Geometry: see drawing. Coordinates: mm, zero at the bounding-box minimum. A direction names the side the tool comes from. Coordinates: 2 decimals unless noted, no trailing zeros. Write each loop counter-clockwise with the first axis right and the second up, starting at its lowest first coordinate (ties: lowest second). Pieces come first, ordered by that corner, then holes. Notation, with made-up numbers: (-21, 9) - (-10, 9) arc R22 ccw to (-10, 41) - close; hole circle Ø9 at (12.5, -24.75). An arc over 180 degrees is marked (long way). One line per question, with ' | ' between items. Start each with the question number.
Q1. Contact query for flat-ended pins moving along their axis: P1, Ø2, axis at x = 5.5, z = 34, coming from the -Y side; P2, Ø1, axis at y = 4.5, z = 10, coming from the -X side. Output: stop coordinate, or through.
Q2. Cut plane A-A, the plane z = 9.5. Return loops of the section in (x, y).
Q3. Line query: line 1 (Z direction, x = 6.5, y = 2.25); line 2 (Y direction, x = 4.5, z = 2); line 3 (Y direction, x = 5, z = 3) (1 decimal). Output: solid intervals per line, ascending.
Q4. Access query for the marked faces 1 and 2. Directions: +Z, -Z, +X, -X, +Y, -Y. A direction counts if a zero-diameter tool reaches every point of the face in a straight line with its end or side. Return the directions, or none.
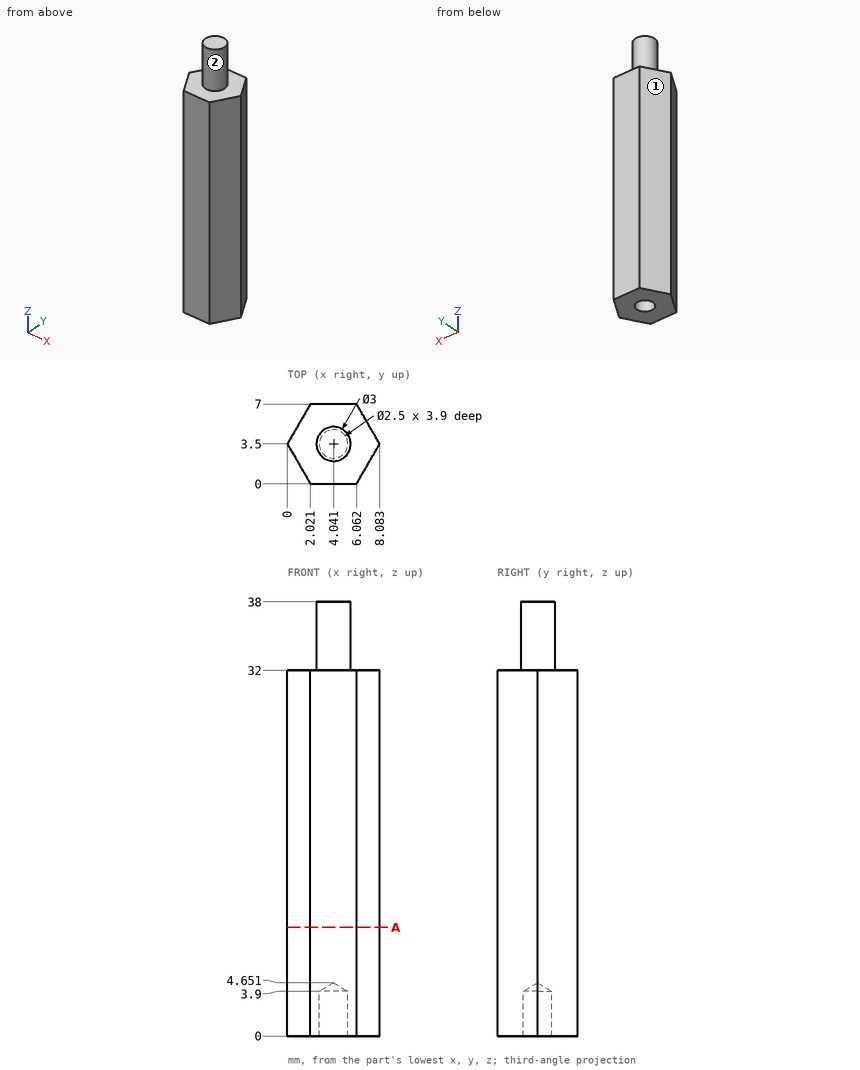
Reply:
1) P1: stops at y = 2.07 | P2: stops at x = 0.29
2) outline: (0, 3.5) - (2.02, 0) - (6.06, 0) - (8.08, 3.5) - (6.06, 7) - (2.02, 7) - close
3) line 1: z = 0 to 32 | line 2: y = 0 to 2.34, 4.66 to 7 | line 3: y = 0 to 2.7, 4.3 to 7
4) face 1: +Z, -Z, -X, +Y | face 2: +Z
